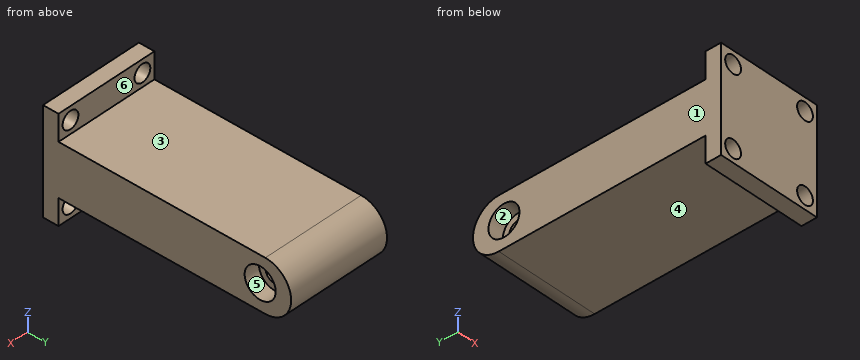
```python
from build123d import *

# Parameters (mm, degrees)
SKETCH1_W           = 20
SKETCH1_H           = 20
BOSS_EXTRUDE1_DEPTH = 52
SKETCH2_R           = 3
CUT_EXTRUDE1_DEPTH  = 3
SKETCH3_R           = 1.75
CUT_EXTRUDE2_DEPTH  = 56.614746246
CUT_EXTRUDE3_START  = -3
SKETCH4_R           = 3
CUT_EXTRUDE3_DEPTH  = 3
SKETCH5_R           = 1.649559613
CUT_EXTRUDE4_DEPTH  = 54.888774341
CUT_EXTRUDE5_DEPTH  = 57.603886792


with BuildPart() as part:
    # Sketch1 → Boss-Extrude1 (new body)
    with BuildSketch(Plane(origin=(0, 0, 0), x_dir=(1, 0, 0), z_dir=(0, 1, 0))):
        Rectangle(SKETCH1_W, SKETCH1_H)
    extrude(amount=BOSS_EXTRUDE1_DEPTH)

    # Sketch2 → Cut-Extrude1 (cut)
    with BuildSketch(Plane(origin=(10, 0, 0), x_dir=(0, 0, -1), z_dir=(1, 0, 0))):
        with Locations((0, 42)):
            Circle(SKETCH2_R)
    extrude(amount=-CUT_EXTRUDE1_DEPTH, mode=Mode.SUBTRACT)

    # Sketch3 → Cut-Extrude2 (cut, through all)
    with BuildSketch(Plane(origin=(7, 0, 0), x_dir=(0, 0, -1), z_dir=(1, 0, 0))):
        with Locations((0, 42)):
            Circle(SKETCH3_R)
    extrude(amount=-CUT_EXTRUDE2_DEPTH, mode=Mode.SUBTRACT)

    # Sketch4 → Cut-Extrude3 (cut)
    with BuildSketch(Plane.ZY.offset(10).offset(CUT_EXTRUDE3_START)):
        with Locations(Location((0, 42, 0), (0, 0, 180))):
            Circle(SKETCH4_R)
    extrude(amount=CUT_EXTRUDE3_DEPTH, mode=Mode.SUBTRACT)

    # Sketch5 → Cut-Extrude4 (cut, through all)
    with BuildSketch(Plane(origin=(0, 52, 0), x_dir=(1, 0, 0), z_dir=(0, 1, 0))):
        with Locations(Location((-7.5, 7.5, 0), (0, 0, 270))):
            Circle(SKETCH5_R)
        with Locations(Location((7.5, 7.5, 0), (0, 0, 270))):
            Circle(SKETCH5_R)
        with Locations(Location((7.5, -7.5, 0), (0, 0, 270))):
            Circle(SKETCH5_R)
        with Locations(Location((-7.5, -7.5, 0), (0, 0, 270))):
            Circle(SKETCH5_R)
    extrude(amount=-CUT_EXTRUDE4_DEPTH, mode=Mode.SUBTRACT)

    # Sketch6 → Cut-Extrude5 (cut, through all)
    with BuildSketch(Plane.ZY.offset(10)):
        with BuildLine():
            Line((-10, 3), (-5, 3))
            Line((-5, 3), (-5, 43))
            ThreePointArc((-5, 43), (0, 48), (5, 43))
            Line((5, 43), (5, 3))
            Line((5, 3), (10, 3))
            Line((10, 3), (10, 52))
            Line((10, 52), (-10, 52))
            Line((-10, 52), (-10, 3))
        make_face()
    extrude(amount=-CUT_EXTRUDE5_DEPTH, mode=Mode.SUBTRACT)


solid = part.part
```
Could you check a few things on this model? Use its own coordinates, in mm. Face numbers are marked on the shaded views. A direction names the side the tool comes from. Coordinates: 2 decimals unless noted, no trailing zeros. Write each loop counter-clockwise with the first axis right and the second up, starting at its lowest first coordinate (ties: lowest second). Pieces come first, ordered by that corner, then holes. Notation, with made-up numbers: (-16.75, 69.5) -> (4.25, 69.5) arc R32 cw to (4.25, 102.5) -> close; hole circle Ø5 at (-12, -32). An arc over 180 degrees is marked (long way). Return JSON: item names as keys, results as strings.
(1) Which directions (+Z, -Z, +X, -X, +Y, -Y) give clear straight access to the entire face, cutting with the end or side of a thin tool? Please do the marked faces 1, 2 and 3.
Numbers:
{"face 1": "+Z, -Z, -X, +Y, -Y", "face 2": "-X", "face 3": "+Z, +X, -X, +Y"}
(2) Imagine slicing it at A-A, the plane x = -7.5. Please give me the cut outline in (y, z), then the cut area to 3 significant figures.
Numbers:
{"outline": "(0, -10) -> (3, -10) -> (3, -9.15) -> (0, -9.15) -> close; (0, -5.85) -> (3, -5.85) -> (3, -5) -> (43, -5) arc R5 ccw to (43, 5) -> (3, 5) -> (3, 5.85) -> (0, 5.85) -> close; (0, 9.15) -> (3, 9.15) -> (3, 10) -> (0, 10) -> close; hole circle Ø6 at (42, 0)", "area": "451 mm2"}
(3) Imagine slicing it at C-C, the plane z = -7.5. Please give me the cut outline in (x, y).
Numbers:
{"outline": "(-10, 0) -> (-9.15, 0) -> (-9.15, 3) -> (-10, 3) -> close; (-5.85, 0) -> (5.85, 0) -> (5.85, 3) -> (-5.85, 3) -> close; (9.15, 0) -> (10, 0) -> (10, 3) -> (9.15, 3) -> close"}
(4) I need wall thicknesses on L1, parallel to X at y = 1.15, z = -7.5; L2, parallel to Y at x = 0.5, z = 0; L3, parallel to Y at x = -8.8, z = 0. Which ranges of each line are inside material? Lowest first, please.
Numbers:
{"L1": "x = -10 to -9.15, -5.85 to 5.85, 9.15 to 10", "L2": "y = 0 to 40.25, 43.75 to 48", "L3": "y = 0 to 39, 45 to 48"}
(5) We'd pull the mould along Z, two halves only. Please class the marked faces 4, 5 and 6: +Z half, -Z half, draft (parallel to the pull), parting line (faces both ways), or undercut.
Numbers:
{"face 4": "-Z half", "face 5": "undercut", "face 6": "draft"}
(6) Imagine slicing it at B-B, the plane y = 42. Please give me the cut outline in (x, z), then the cut area to 3 significant figures.
Numbers:
{"outline": "(-10, -5) -> (10, -5) -> (10, -3) -> (7, -3) -> (7, -1.75) -> (-7, -1.75) -> (-7, -3) -> (-10, -3) -> close; (-10, 3) -> (-7, 3) -> (-7, 1.75) -> (7, 1.75) -> (7, 3) -> (10, 3) -> (10, 5) -> (-10, 5) -> close", "area": "115 mm2"}
(7) Imagine slicing it at D-D, the plane z = 0. Please give me the cut outline in (x, y), then the cut area to 3 significant figures.
Numbers:
{"outline": "(-10, 0) -> (10, 0) -> (10, 39) -> (7, 39) -> (7, 40.25) -> (-7, 40.25) -> (-7, 39) -> (-10, 39) -> close; (-10, 45) -> (-7, 45) -> (-7, 43.75) -> (7, 43.75) -> (7, 45) -> (10, 45) -> (10, 48) -> (-10, 48) -> close", "area": "875 mm2"}
(8) I'm going to push flat-ended pins straight in: pin 1 (5.5 mm diameter, centred on x = 1.5, z = 6.5, fed in from +Y); pin 2 (1 mm diameter, centred on x = 5.5, z = -8, fed in from +Y); pin 3 (10 mm diameter, centred on x = -2.5, y = 29, fed in from -Z); pin 4 (3 mm diameter, centred on x = -7.5, z = 7.5, fed in from -Y). Where does each tip first touch, or does it pass through?
Numbers:
{"pin 1": "stops at y = 46.31", "pin 2": "stops at y = 3", "pin 3": "stops at z = -5", "pin 4": "passes through"}
